Geometry: see drawing. Coordinates: mm, zero at the bounding-box minimum. Give positions to 0.01 mm unless a question says otherwise; leave off trailing zeros. Loops run counter-clockwise (first coordinate to the right, second up) from the corner with the lowest first, then second, coordinate; pieces in that order, holes last. Notation, with made-up numbers: (57.5, 77) -> (110.5, 77) arc R17 ccw to (110.5, 84) -> close; hole circle Ø5 at (-37, 44.25). An arc over 180 degrees is marked (long way). Use CSV: the item, a comma, the result in double quotes.
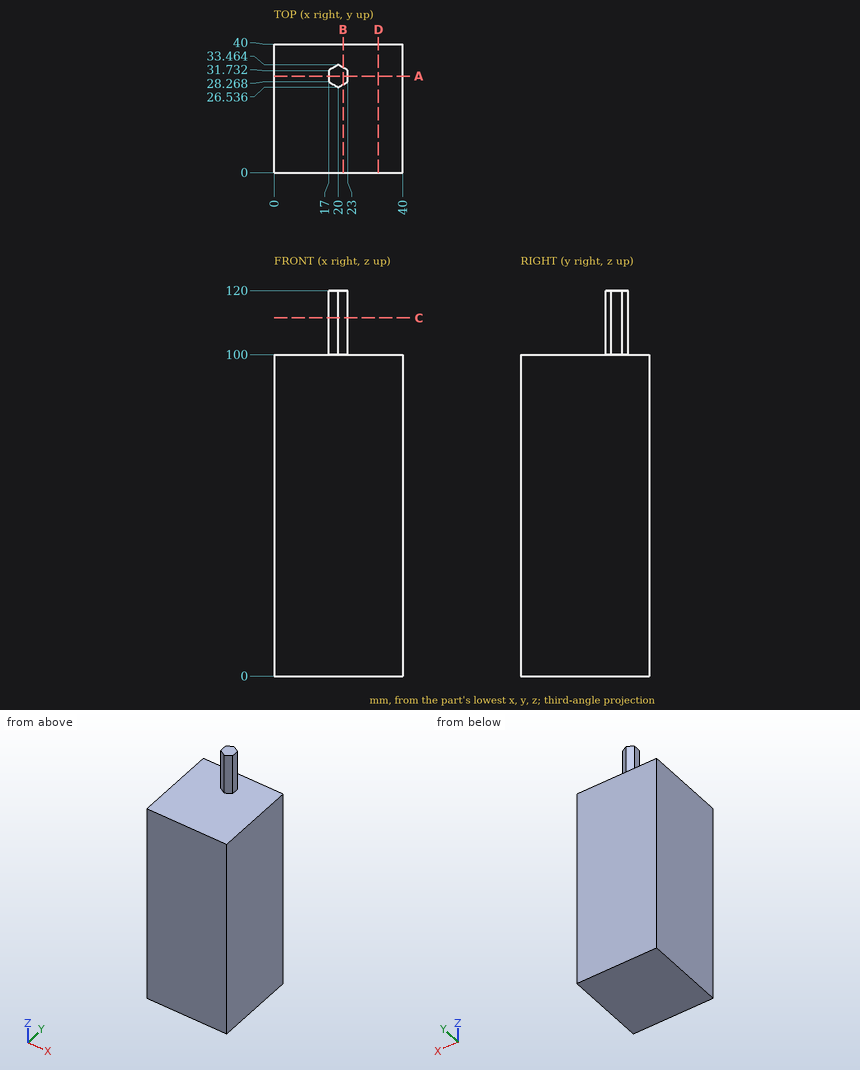
1) Section query C-C (z = 111.5). Return loops of the section in (x, y).
From the geometry:
outline,"(17, 28.27) -> (20, 26.54) -> (23, 28.27) -> (23, 31.73) -> (20, 33.46) -> (17, 31.73) -> close"
2) Contact query for flat-ended pins moving along their axis: pin 1 (1.5 mm diameter, centred on x = 34, y = 10.5, fed in from +Z); pin 2 (1.7 mm diameter, centred on y = 29, z = 114, fed in from -X); pin 3 (3 mm diameter, centred on x = 14, y = 17, fed in from -Z); pin 4 (1 mm diameter, centred on y = 29.5, z = 112, fed in from +X). Output: stop coordinate, or through.
From the geometry:
pin 1,"stops at z = 100"
pin 2,"stops at x = 17"
pin 3,"stops at z = 0"
pin 4,"stops at x = 23"
3) Ray query, line 1 (Z direction, x = 13, y = 34.5). Return the intervals inside material, ascending.
From the geometry:
line 1,"z = 0 to 100"
4) Section query A-A (y = 30). Return loops of the section in (x, z).
From the geometry:
outline,"(0, 0) -> (40, 0) -> (40, 100) -> (23, 100) -> (23, 120) -> (17, 120) -> (17, 100) -> (0, 100) -> close"
5) Section query B-B (x = 21.5). Return loops of the section in (y, z).
From the geometry:
outline,"(0, 0) -> (40, 0) -> (40, 100) -> (32.6, 100) -> (32.6, 120) -> (27.4, 120) -> (27.4, 100) -> (0, 100) -> close"
6) Section query D-D (x = 32.5). Return loops of the section in (y, z), then the cut area to 3 significant figures.
From the geometry:
outline,"(0, 0) -> (40, 0) -> (40, 100) -> (0, 100) -> close"
area,"4,000 mm^2"
